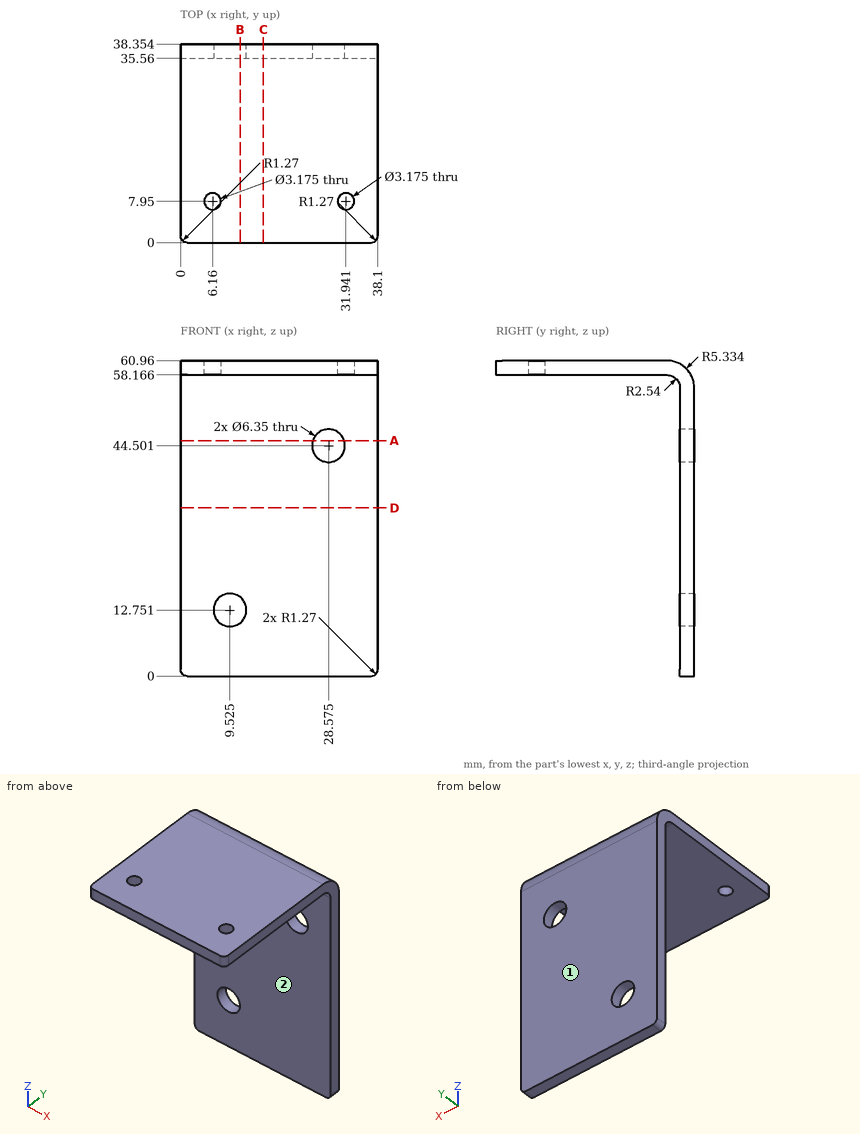
Source: three-view drawing plus pictorial views. Frame: mm from the lowest corner of the part. A direction names the side the tool comes from. Round coordinates to 2 decimals unless told otherwise and drop trailing zeros. Loops run counter-clockwise (first coordinate to the right, second up) from the corner with the lowest first, then second, coordinate; pieces in that order, holes last.
Q1. Section C-C, the plane x = 16. Return loops of the section in (y, z) (1 decimal).
Q2. Access query for the marked faces 1 and 2. Directions: +Z, -Z, +X, -X, +Y, -Y. A direction counts if a zero-diameter tool reaches every point of the face in a straight line with its end or side. Return the directions, or none.
Q3. Section D-D, the plane z = 32.5. Return loops of the section in (x, y) (1 decimal).
Q4. Section A-A, the plane z = 45.5. Return loops of the section in (x, y) (1 decimal).
Q5. First-contact query: P1, Ø12, axis at x = 17, y = 32.5, coming from the -Z side; P2, Ø12, axis at x = 17, z = 38, coming from the -Y side. Flat tips, straight axial feed; report the tip coordinate or a pass-through.
Q6. Ray query, line 1 (Z direction, x = 6, y = 17.5) (1 decimal); line 2 (Y direction, x = 17, z = 14) (1 decimal); line 3 (Z direction, x = 10.5, y = 34). Return the intervals inside material, ascending.
Q7. Section B-B, the plane x = 11.5. Return loops of the section in (y, z) (1 decimal).
Solutions:
1. outline: (0, 58.2) - (33, 58.2) arc R2.5 cw to (35.6, 55.6) - (35.6, 0) - (38.4, 0) - (38.4, 55.6) arc R5.3 ccw to (33, 61) - (0, 61) - close
2. face 1: +Z, -Z, +X, -X, +Y
2. face 2: -Z, +X, -X, -Y
3. outline: (0, 35.6) - (38.1, 35.6) - (38.1, 38.4) - (0, 38.4) - close
4. outline: (0, 35.6) - (25.6, 35.6) - (25.6, 38.4) - (0, 38.4) - close; (31.6, 35.6) - (38.1, 35.6) - (38.1, 38.4) - (31.6, 38.4) - close
5. P1: stops at z = 0
5. P2: stops at y = 35.56
6. line 1: z = 58.2 to 61
6. line 2: y = 35.6 to 38.4
6. line 3: z = 57.97 to 60.87
7. outline: (0, 58.2) - (33, 58.2) arc R2.5 cw to (35.6, 55.6) - (35.6, 15.2) - (38.4, 15.2) - (38.4, 55.6) arc R5.3 ccw to (33, 61) - (0, 61) - close; (35.6, 0) - (38.4, 0) - (38.4, 10.3) - (35.6, 10.3) - close
